Geometry: see drawing. Coordinates: mm, zero at the bounding-box minimum. A direction names the side the tool comes from. Give positions to 0.01 mm unless a question says otherwise; leave off trailing zeros. Loops run counter-clockwise (first coordinate to the right, second up) from the corner with the lowest first, then second, coordinate; pieces in that order, holes last. Notation, with made-up numbers: (47, 30.25) -> (95, 30.25) arc R20 ccw to (95, 50.25) -> close; hole circle Ø7 at (75.5, -29). An arc over 180 degrees is marked (long way). One line per question, with ' | ' between items.
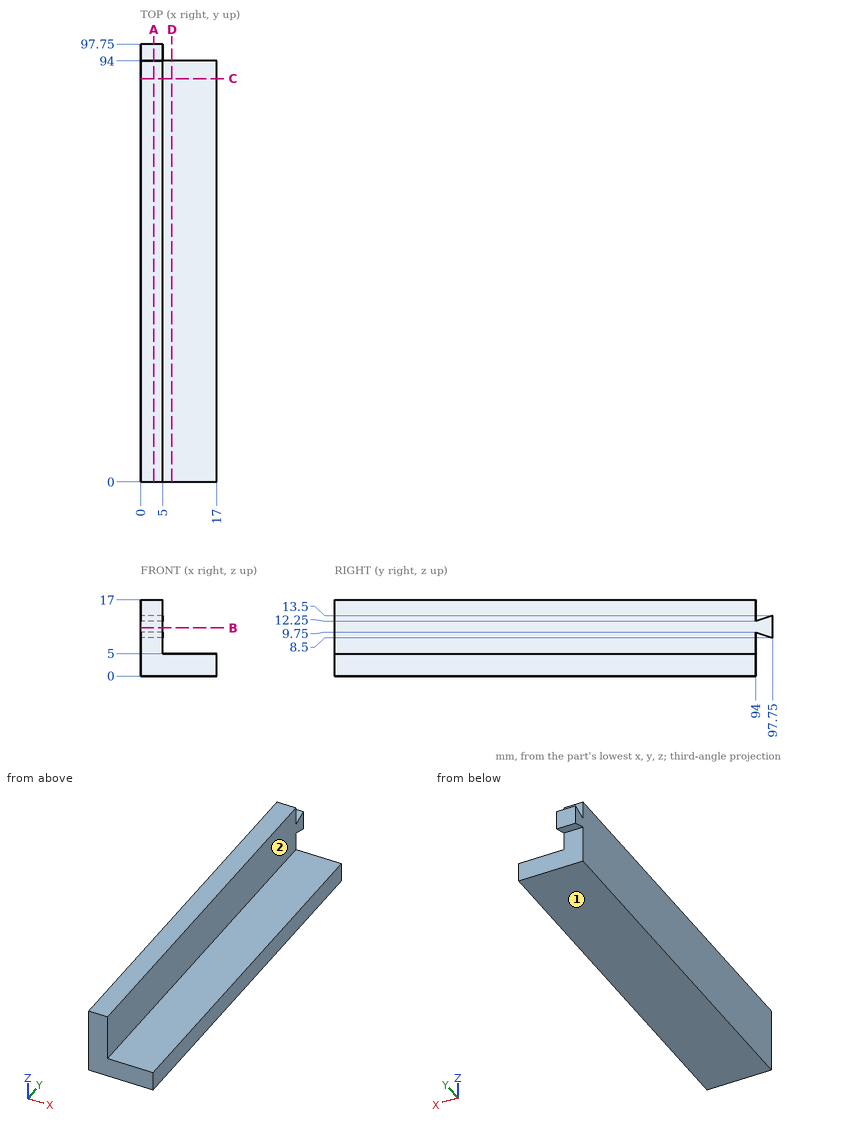
1. Section query C-C (y = 90). Output: boundary loops of the cut face in (x, z).
Determined:
outline: (0, 0) -> (17, 0) -> (17, 5) -> (5, 5) -> (5, 17) -> (0, 17) -> close
2. Reachability of the marked faces 1 and 2 from +Z, -Z, +X, -X, +Y, -Y: full face, straight path, thin tool, end or side. Return the list, or none.
Determined:
face 1: -Z, +X, -X, +Y, -Y | face 2: +Z, +X, +Y, -Y
3. Section query A-A (x = 3). Output: boundary loops of the cut face in (y, z).
Determined:
outline: (0, 0) -> (94, 0) -> (94, 9.75) -> (97.75, 8.5) -> (97.75, 13.5) -> (94, 12.25) -> (94, 17) -> (0, 17) -> close
4. Section query B-B (z = 10.75). Output: boundary loops of the cut face in (x, y), then the cut area to 3 significant figures.
Determined:
outline: (0, 0) -> (5, 0) -> (5, 97.75) -> (0, 97.75) -> close | area: 489 mm2
5. Pin query (flat end, axial travel): P1, Ø3.5, axis at x = 8.5, y = 55, coming from the +Z side. Return the tip coordinate at first contact, or that it passes through.
Determined:
P1: stops at z = 5
6. Section query D-D (x = 7). Output: boundary loops of the cut face in (y, z).
Determined:
outline: (0, 0) -> (94, 0) -> (94, 5) -> (0, 5) -> close
7. Ray query, line 1 along Y through (x, z) = (3.5, 8); line 2 along Z through (x, y) = (15.25, 25.5). Return the intervals inside material, ascending. Write a range as from..to.
Determined:
line 1: y = 0..94 | line 2: z = 0..5
